```python
from build123d import *
from build123d.topology import SkipClean

# Parameters (mm, degrees)
SKETCH1_R           = 4.3
SKETCH1_R_2         = 2.8
SKETCH1_W           = 5
SKETCH1_H           = 2
BOSS_EXTRUDE1_DEPTH = 5.5
SKETCH2_R           = 2.8
BOSS_EXTRUDE2_DEPTH = 2.5
SKETCH3_W           = 5
SKETCH3_H           = 2
SKETCH3_H_2         = 1.945877
BOSS_EXTRUDE3_DEPTH = 1.8
SKETCH4_RX          = 2.5
SKETCH4_RY          = 1.945877
BOSS_EXTRUDE4_DEPTH = 2
CUT_EXTRUDE1_REACH  = 116.662
BOSS_EXTRUDE5_DEPTH = 2.5
SKETCH7_R           = 1.75
CUT_EXTRUDE2_DEPTH  = 115.431852156
CUT_EXTRUDE3_DEPTH  = 12.446


with BuildPart() as part:
    # Sketch1 → Boss-Extrude1 (new body)
    # profile 1 of 6: a face of its own
    with BuildSketch(Plane.XY):
        with Locations((-96.304, 4.712)):
            Circle(SKETCH1_R)
        with Locations((-96.304, 4.712)):
            Circle(SKETCH1_R_2, mode=Mode.SUBTRACT)
    # profile 2 of 6: a face of its own
    with BuildSketch(Plane.XY):
        with Locations((-39.408, 4.712)):
            Circle(SKETCH1_R)
        with Locations((-39.408, 4.712)):
            Circle(SKETCH1_R_2, mode=Mode.SUBTRACT)
    # profile 3 of 6: a face of its own
    with BuildSketch(Plane.XY):
        with Locations((-98.72988, 49.487957)):
            Rectangle(SKETCH1_W, SKETCH1_H)
    # profile 4 of 6: a face of its own
    with BuildSketch(Plane.XY):
        with Locations((-98.72988, 51.487957)):
            Rectangle(SKETCH1_W, SKETCH1_H)
    # profile 5 of 6: a face of its own
    with BuildSketch(Plane.XY):
        with Locations((-21.198302598, 49.54208)):
            Rectangle(SKETCH1_W, SKETCH1_H)
    # profile 6 of 6: a face of its own
    with BuildSketch(Plane.XY):
        with Locations((-21.198302598, 51.54208)):
            Rectangle(SKETCH1_W, SKETCH1_H)
    extrude(amount=BOSS_EXTRUDE1_DEPTH)

    # Sketch2 → Boss-Extrude2 (add)
    with BuildSketch(Plane.XY.offset(5.5)):
        with BuildLine():
            Line((-96.304, 0.412), (-39.408, 0.412))
            ThreePointArc((-39.408, 0.412), (-35.108, 4.712), (-39.408, 9.012))
            Line((-39.408, 9.012), (-58.798327935, 9.012))
            Line((-58.798327935, 9.012), (-18.698302598, 48.54208))
            Line((-18.698302598, 48.54208), (-18.698302598, 52.54208))
            Line((-18.698302598, 52.54208), (-23.698302598, 52.54208))
            Line((-23.698302598, 52.54208), (-67.856, 9.012))
            Line((-67.856, 9.012), (-96.22988, 52.487957))
            Line((-96.22988, 52.487957), (-101.22988, 52.487957))
            Line((-101.22988, 52.487957), (-101.22988, 48.487957))
            Line((-101.22988, 48.487957), (-75.46653529, 9.012))
            Line((-75.46653529, 9.012), (-96.304, 9.012))
            ThreePointArc((-96.304, 9.012), (-100.604, 4.712), (-96.304, 0.412))
        make_face()
        with Locations((-96.304, 4.712)):
            Circle(SKETCH2_R, mode=Mode.SUBTRACT)
        with Locations((-39.408, 4.712)):
            Circle(SKETCH2_R, mode=Mode.SUBTRACT)
    extrude(amount=BOSS_EXTRUDE2_DEPTH)

    # Sketch3 → Boss-Extrude3 (add)
    with BuildSketch(Plane(origin=(0, 0, 0), x_dir=(-1, 0, 0), z_dir=(0, 0, -1))):
        with Locations((21.198302598, 51.54208)):
            Rectangle(SKETCH3_W, SKETCH3_H)
        with Locations((98.72988, 51.5150185)):
            Rectangle(SKETCH3_W, SKETCH3_H_2)
    extrude(amount=BOSS_EXTRUDE3_DEPTH)

    # Sketch4 → Boss-Extrude4 (add)
    with BuildSketch(Plane(origin=(0, 0, -1.8), x_dir=(-1, 0, 0), z_dir=(0, 0, -1))):
        with BuildLine():
            add(Edge.make_bspline(
                [(101.22988, 50.54208), (101.22988, 52.487957031), (98.72987996, 52.487957)],
                knots=[0, 0, 0, 1.570796343, 1.570796343, 1.570796343], degree=2, weights=[1, 0.707106776, 1]))
            Line((101.22988, 50.54208), (101.22988, 52.487957))
            Line((101.22988, 52.487957), (98.72987996, 52.487957))
        make_face()
        with BuildLine():
            Line((96.22988, 52.487957), (96.22988, 50.54208))
            add(Edge.make_bspline(
                [(98.72987996, 52.487957), (96.22988, 52.487956969), (96.22988, 50.54208)],
                knots=[1.570796343, 1.570796343, 1.570796343, 3.141592654, 3.141592654, 3.141592654], degree=2, weights=[1, 0.707106787, 1]))
            Line((98.72987996, 52.487957), (96.22988, 52.487957))
        make_face()
        with Locations((98.72988, 50.54208)):
            Ellipse(SKETCH4_RX, SKETCH4_RY)
        with BuildLine():
            Line((18.698302598, 52.54208), (18.698302598, 50.54208))
            add(Edge.make_bspline(
                [(21.198302598, 52.54208), (18.698302598, 52.54208), (18.698302598, 50.54208)],
                knots=[1.570796327, 1.570796327, 1.570796327, 3.141592654, 3.141592654, 3.141592654], degree=2, weights=[1, 0.707106781, 1]))
            Line((21.198302598, 52.54208), (18.698302598, 52.54208))
        make_face()
        with BuildLine():
            add(Edge.make_bspline(
                [(23.698302598, 50.54208), (23.698302598, 52.54208), (21.198302598, 52.54208)],
                knots=[0, 0, 0, 1.570796327, 1.570796327, 1.570796327], degree=2, weights=[1, 0.707106781, 1]))
            Line((23.698302598, 50.54208), (23.698302598, 52.54208))
            Line((23.698302598, 52.54208), (21.198302598, 52.54208))
        make_face()
        with BuildLine():
            Line((23.698302598, 50.54208), (18.698302598, 50.54208))
            add(Edge.make_bspline(
                [(18.698302598, 50.54208), (18.698302598, 48.54208), (21.198302598, 48.54208), (23.698302598, 48.54208), (23.698302598, 50.54208)],
                knots=[3.141592654, 3.141592654, 3.141592654, 4.71238898, 4.71238898, 6.283185307, 6.283185307, 6.283185307], degree=2, weights=[1, 0.707106781, 1, 0.707106781, 1]))
        make_face()
        with BuildLine():
            add(Edge.make_bspline(
                [(21.198302598, 52.54208), (18.698302598, 52.54208), (18.698302598, 50.54208)],
                knots=[1.570796327, 1.570796327, 1.570796327, 3.141592654, 3.141592654, 3.141592654], degree=2, weights=[1, 0.707106781, 1]))
            Line((18.698302598, 50.54208), (23.698302598, 50.54208))
            add(Edge.make_bspline(
                [(23.698302598, 50.54208), (23.698302598, 52.54208), (21.198302598, 52.54208)],
                knots=[0, 0, 0, 1.570796327, 1.570796327, 1.570796327], degree=2, weights=[1, 0.707106781, 1]))
        make_face()
        with BuildLine():
            Line((23.698302598, 50.54208), (18.698302598, 50.54208))
            add(Edge.make_bspline(
                [(18.698302598, 50.54208), (18.698302598, 48.54208), (21.198302598, 48.54208), (23.698302598, 48.54208), (23.698302598, 50.54208)],
                knots=[3.141592654, 3.141592654, 3.141592654, 4.71238898, 4.71238898, 6.283185307, 6.283185307, 6.283185307], degree=2, weights=[1, 0.707106781, 1, 0.707106781, 1]))
        make_face()
        with BuildLine():
            add(Edge.make_bspline(
                [(21.198302598, 52.54208), (18.698302598, 52.54208), (18.698302598, 50.54208)],
                knots=[1.570796327, 1.570796327, 1.570796327, 3.141592654, 3.141592654, 3.141592654], degree=2, weights=[1, 0.707106781, 1]))
            Line((18.698302598, 50.54208), (23.698302598, 50.54208))
            add(Edge.make_bspline(
                [(23.698302598, 50.54208), (23.698302598, 52.54208), (21.198302598, 52.54208)],
                knots=[0, 0, 0, 1.570796327, 1.570796327, 1.570796327], degree=2, weights=[1, 0.707106781, 1]))
        make_face()
    extrude(amount=BOSS_EXTRUDE4_DEPTH)

    # Sketch5 → Cut-Extrude1 (cut, up to next)
    with BuildSketch(Plane.XY.offset(8), mode=Mode.PRIVATE) as cut_extrude1_sk1:
        with BuildLine():
            ThreePointArc((-78.201246925, 4.712), (-76.451246925, 2.962), (-74.701246925, 4.712))
            Line((-74.701246925, 4.712), (-78.201246925, 4.712))
        make_face()
    cut_extrude1_tool1 = extrude(cut_extrude1_sk1.sketch, amount=-CUT_EXTRUDE1_REACH, mode=Mode.PRIVATE) & part.part
    # Sketch5 → Cut-Extrude1 (cut, up to next)
    with BuildSketch(Plane.XY.offset(8), mode=Mode.PRIVATE) as cut_extrude1_sk2:
        with BuildLine():
            Line((-78.201246925, 4.712), (-74.701246925, 4.712))
            ThreePointArc((-74.701246925, 4.712), (-76.451246925, 6.462), (-78.201246925, 4.712))
        make_face()
    cut_extrude1_tool2 = extrude(cut_extrude1_sk2.sketch, amount=-CUT_EXTRUDE1_REACH, mode=Mode.PRIVATE) & part.part
    # Sketch5 → Cut-Extrude1 (cut, up to next)
    with BuildSketch(Plane.XY.offset(8), mode=Mode.PRIVATE) as cut_extrude1_sk3:
        with BuildLine():
            ThreePointArc((-78.201246925, 4.712), (-76.451246925, 2.962), (-74.701246925, 4.712))
            Line((-74.701246925, 4.712), (-78.201246925, 4.712))
        make_face()
    cut_extrude1_tool3 = extrude(cut_extrude1_sk3.sketch, amount=-CUT_EXTRUDE1_REACH, mode=Mode.PRIVATE) & part.part
    # Sketch5 → Cut-Extrude1 (cut, up to next)
    with BuildSketch(Plane.XY.offset(8), mode=Mode.PRIVATE) as cut_extrude1_sk4:
        with BuildLine():
            Line((-78.201246925, 4.712), (-74.701246925, 4.712))
            ThreePointArc((-74.701246925, 4.712), (-76.451246925, 6.462), (-78.201246925, 4.712))
        make_face()
    cut_extrude1_tool4 = extrude(cut_extrude1_sk4.sketch, amount=-CUT_EXTRUDE1_REACH, mode=Mode.PRIVATE) & part.part
    add(cut_extrude1_tool1.solids().sort_by_distance((-76.451247, 3.969277, 8))[0], mode=Mode.SUBTRACT)
    add(cut_extrude1_tool2.solids().sort_by_distance((-76.451247, 5.454723, 8))[0], mode=Mode.SUBTRACT)
    add(cut_extrude1_tool3.solids().sort_by_distance((-76.451247, 3.969277, 8))[0], mode=Mode.SUBTRACT)
    add(cut_extrude1_tool4.solids().sort_by_distance((-76.451247, 5.454723, 8))[0], mode=Mode.SUBTRACT)

    # Sketch6 → Boss-Extrude5 (add, through all)
    with BuildSketch(Plane(origin=(0, 0, 5.5), x_dir=(-1, 0, 0), z_dir=(0, 0, -1))):
        with BuildLine():
            Line((52.194141657, 24.451254914), (52.578584331, 24.780782125))
            ThreePointArc((52.578584331, 24.780782125), (52.86162294, 28.845811152), (48.792917769, 29.069887196))
            Line((48.792917769, 29.069887196), (45.000367772, 31.542783031))
            Line((45.000367772, 31.542783031), (49.066381254, 27.534560172))
            ThreePointArc((49.066381254, 27.534560172), (51.011962302, 28.67771538), (52.466845, 26.952778923))
            ThreePointArc((52.466845, 26.952778923), (52.152438331, 25.951993337), (51.322191527, 25.310811938))
            Line((51.322191527, 25.310811938), (52.194141657, 24.451254914))
        make_face()
    extrude(amount=-BOSS_EXTRUDE5_DEPTH)

    # Sketch7 → Cut-Extrude2 (cut, through all)
    with BuildSketch(Plane(origin=(0, 0, 5.5), x_dir=(-1, 0, 0), z_dir=(0, 0, -1))):
        with Locations((51.451246925, 4.712)):
            Circle(SKETCH7_R)
    extrude(amount=-CUT_EXTRUDE2_DEPTH, mode=Mode.SUBTRACT)

    # Sketch6<3> → Cut-Extrude3 (cut)
    with SkipClean():  # the faces are left unmerged after this step: merging them gives an invalid solid
        with BuildSketch(Plane(origin=(0, 0, 5.5), x_dir=(-1, 0, 0), z_dir=(0, 0, -1))):
            with BuildLine():
                ThreePointArc((49.066381254, 27.534560172), (49.488296444, 25.706517135), (51.322191527, 25.310811938))
                Line((51.322191527, 25.310811938), (49.066381254, 27.534560172))
            make_face()
            with BuildLine():
                Line((49.066381254, 27.534560172), (51.322191527, 25.310811938))
                ThreePointArc((51.322191527, 25.310811938), (52.152438331, 25.951993337), (52.466845, 26.952778923))
                ThreePointArc((52.466845, 26.952778923), (51.011962302, 28.67771538), (49.066381254, 27.534560172))
            make_face()
        extrude(amount=-CUT_EXTRUDE3_DEPTH, mode=Mode.SUBTRACT)


solid = part.part
```
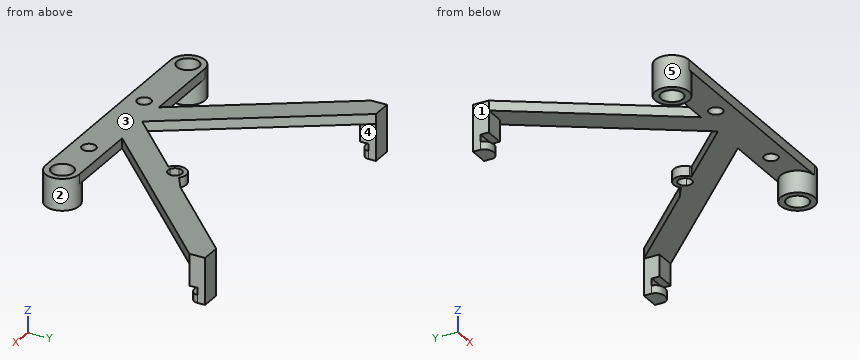
Model file for the job. Use its own axes, mm. Face numbers are marked on the shaded views. A direction names the side the tool comes from. Round coordinates to 2 decimals unless told otherwise and drop trailing zeros. Loops run counter-clockwise (first coordinate to the right, second up) from the corner with the lowest first, then second, coordinate; pieces in that order, holes last. Notation, with made-up numbers: M 55.25,64.5 L 108.25,64.5 A30 cw 108.25,103.5 Z; hole C -30,5.25 d4. An arc over 180 degrees is marked long. Put each result on its own line as item: value. Start each with the question number.
Item 1: 3-axis set-ups, long thin cutter, end or side, ignore diameter. For the marked faces 4 and 5: which of +Z, -Z, +X, -X, +Y, -Y reach the whole face in a straight line?
Item 2: Mould opens along X. For the marked faces 1, 2 and 3 say: released by +X, released by -X, zero draft, split by the parting line, or undercut.
Item 3: Cut at B-B (y = 20.5). List the corners of the cut face in (x, z), then the cut area to 3 significant figures.
Item 4: Drill centre lines: line 1 along Y through (x, z) = (-53, 5.75); line 2 along Z through (x, y) = (-74, 13); line 3 along Y through (x, z) = (-90, 6.75). Where is each one in solid material? Low to high.
Item 5: Drop flat-ended pins along their axis: P1, Ø1.5, axis at x = -99.5, z = 4.5, coming from the +Y side; P2, Ø0.9, axis at x = -20.5, z = -1, coming from the -Y side; P3, Ø4, axis at x = -21, z = 4, coming from the -Y side. Give the stop position or say it passes through.
Item 6: Cut at D-D (x = -41). List the corners of the cut face in (y, z).
Item 7: Cut at A-A (z = 2.75). List the corners of the cut face in (x, y).
Item 8: Cut at C-C (x = -56.5). List the corners of the cut face in (y, z), then the cut area to 3 significant figures.
Answer block:
1. face 4: -Z, +Y
1. face 5: -Z
2. face 1: released by -X
2. face 2: undercut
2. face 3: zero draft
3. outline: M -82.96,5.5 L -75.35,5.5 L -75.35,8 L -82.96,8 Z; M -56.2,5.5 L -47.14,5.5 L -47.14,8 L -56.2,8 Z
3. area: 41.7 mm2
4. line 1: 0.41 to 3.9, 5.53 to 9.01, 14.73 to 23.66, 25.23 to 28.68
4. line 2: 5.5 to 8
4. line 3: 0.41 to 9.01, 31.28 to 42.94
5. P1: y = 52.49
5. P2: y = 50.54
5. P3: y = 44.97
6. outline: M 0.41,5.5 L 0.72,5.5 L 0.72,0 L 2.41,0 L 2.41,8 L 0.41,8 Z; M 7.02,0 L 8.71,0 L 8.71,5.5 L 9.01,5.5 L 9.01,8 L 7.02,8 Z; M 26.56,5.5 L 35.49,5.5 L 35.49,8 L 26.56,8 Z
7. outline: M -101.23,48.49 L -96.23,48.49 L -96.23,52.49 L -101.23,52.49 Z; C -96.3,4.71 d8.6; C -39.41,4.71 d8.6; M -23.7,48.54 L -18.7,48.54 L -18.7,52.54 L -23.7,52.54 Z; hole C -96.3,4.71 d5.6; hole C -39.41,4.71 d5.6
8. outline: M 0.41,5.5 L 9.01,5.5 L 9.01,8 L 0.41,8 Z; M 11.28,5.5 L 20.21,5.5 L 20.21,8 L 11.28,8 Z
8. area: 43.8 mm2
